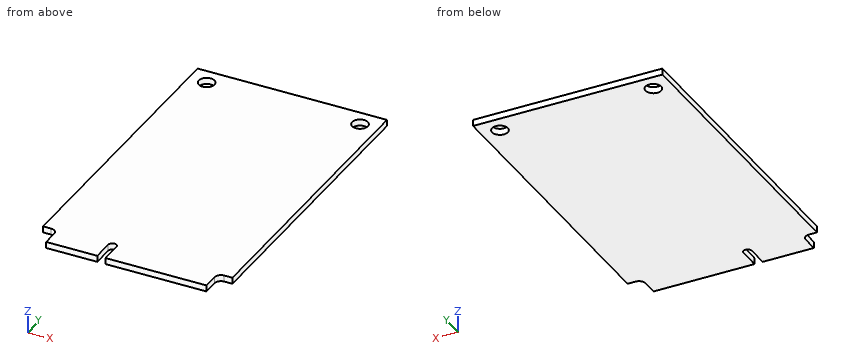
from build123d import *

# Parameters (mm, degrees)
PAD_DEPTH    = 1
SKETCH001_R  = 1.25
POCKET_DEPTH = 1.001


with BuildPart() as part:
    # Sketch → Pad (new body)
    with BuildSketch(Plane.XY):
        with BuildLine():
            Line((-15, -22), (-15, 25.5))
            Line((-15, 25.5), (15, 25.5))
            Line((15, 25.5), (15, -22))
            Line((15, -22), (13.7, -22))
            ThreePointArc((13.7, -22), (12.992893, -22.292893), (12.7, -23))
            Line((12.7, -23), (12.7, -25.5))
            Line((12.7, -25.5), (-3.3, -25.5))
            Line((-3.3, -25.5), (-3.3, -22.15))
            ThreePointArc((-3.3, -22.15), (-3.95, -21.5), (-4.6, -22.15))
            Line((-4.6, -25.5), (-4.6, -22.15))
            Line((-12.7, -25.5), (-4.6, -25.5))
            Line((-12.7, -23), (-12.7, -25.5))
            ThreePointArc((-12.7, -23), (-12.992893, -22.292893), (-13.7, -22))
            Line((-15, -22), (-13.7, -22))
        make_face()
    extrude(amount=PAD_DEPTH)

    # Sketch001 (on Face16 of Pad) → Pocket (cut, through all)
    with BuildSketch(Plane.XY.offset(1)):
        with Locations((-12.15, 22.75)):
            Circle(SKETCH001_R)
        with Locations((12.15, 22.75)):
            Circle(SKETCH001_R)
    extrude(amount=-POCKET_DEPTH, mode=Mode.SUBTRACT)


solid = part.part
The listing builds one solid part. Answer for the finished solid, in the listing's coordinates (mm). Give positions to 0.01 mm unless a question says otherwise; leave off trailing zeros. Write each loop counter-clockwise with the first axis right and the second up, starting at its lowest first coordinate (ties: lowest second). Pieces come first, ordered by that corner, then holes. Notation, with made-up numbers: (-15, 0.25) -> (12, 0.25) arc R20 cw to (12, 4.25) -> close; hole circle Ø11 at (58.5, 10.5). An arc over 180 degrees is marked (long way). One line per question, with ' | ' between items. Start each with the question number.
1. Find the intervals of material crossed by probe 1 along Y at (x, z) = (-12.15, 0.7); probe 2 along X at (y, z) = (-23, 0.35); probe 3 along Y at (x, z) = (-13.25, 0.3), in increasing order.
2. Section B-B (z = 0.6) is taken. Determine the outline of the cut face in (x, y).
3. Section C-C (x = -3.95) is taken. Determine the outline of the cut face in (y, z), plus the area to 3 significant figures.
4. Given pin 1 Ø1.5 at (x, y) = (-12.15, 22.75) entering from +Z; pin 2 Ø0.5 at (x, z) = (14.5, 0.5) entering from -Y, each flat-ended and moving along its own axis, determine where each tip first touches the part or whether it passes through.
5. Section A-A (x = -12.15) is taken. Determine the outline of the cut face in (y, z), plus the area to 3 significant figures.
Response values:
1) probe 1: -25.5 to 21.5, 24 to 25.5 | probe 2: -12.7 to -4.6, -3.3 to 12.7 | probe 3: -22.11 to 22.16, 23.34 to 25.5
2) outline: (-15, -22) -> (-13.7, -22) arc R1 cw to (-12.7, -23) -> (-12.7, -25.5) -> (-4.6, -25.5) -> (-4.6, -22.15) arc R0.65 cw to (-3.3, -22.15) -> (-3.3, -25.5) -> (12.7, -25.5) -> (12.7, -23) arc R1 cw to (13.7, -22) -> (15, -22) -> (15, 25.5) -> (-15, 25.5) -> close; hole circle Ø2.5 at (-12.15, 22.75); hole circle Ø2.5 at (12.15, 22.75)
3) outline: (-21.5, 0) -> (25.5, 0) -> (25.5, 1) -> (-21.5, 1) -> close | area: 47.0 mm2
4) pin 1: through | pin 2: y = -22
5) outline: (-25.5, 0) -> (21.5, 0) -> (21.5, 1) -> (-25.5, 1) -> close; (24, 0) -> (25.5, 0) -> (25.5, 1) -> (24, 1) -> close | area: 48.5 mm2
